from build123d import *

# Parameters (mm, degrees)
SKETCH1_W                = 60
SKETCH1_H                = 50
BOSS_EXTRUDE1_DEPTH      = 10
SKETCH3_W                = 50
SKETCH3_H                = 10
BOSS_EXTRUDE2_DEPTH      = 20
SKETCH2_W                = 20
SKETCH2_H                = 9
CUT_EXTRUDE2_DEPTH       = 2
SKETCH5_W                = 9
SKETCH5_H                = 20.5
CUT_EXTRUDE3_DEPTH       = 2
SKETCH6_R                = 0.75
CUT_EXTRUDE4_DEPTH       = 9
SKETCH9_W                = 10
SKETCH9_H                = 50
BOSS_EXTRUDE3_DEPTH      = 80
FILLET1_R                = 10
FILLET2_R                = 10
FILLET3_R                = 10
FILLET4_R                = 10
FILLET5_R                = 10
SKETCH11_W               = 10.5
SKETCH11_H               = 41
CUT_EXTRUDE5_DEPTH       = 40
SKETCH13_R               = 2
CUT_EXTRUDE6_DEPTH       = 40
MIRROR11_COPY_1_SKETCH_R = 2
MIRROR11_COPY_1_DEPTH    = 40


with BuildPart() as part:
    # Sketch1 → Boss-Extrude1 (new body)
    with BuildSketch(Plane(origin=(0, 0, 0), x_dir=(1, 0, 0), z_dir=(0, 1, 0))):
        with Locations((8.551590838, -18.42193)):
            Rectangle(SKETCH1_W, SKETCH1_H)
    extrude(amount=BOSS_EXTRUDE1_DEPTH)

    # Sketch3 → Boss-Extrude2 (add)
    with BuildSketch(Plane.ZY.offset(21.448409162)):
        with Locations((18.42193, 5)):
            Rectangle(SKETCH3_W, SKETCH3_H)
    extrude(amount=BOSS_EXTRUDE2_DEPTH)

    # Sketch2 → Cut-Extrude2 (cut)
    with BuildSketch(Plane(origin=(0, 10, 0), x_dir=(1, 0, 0), z_dir=(0, 1, 0))):
        with Locations((-18.948409162, -18.42193)):
            Rectangle(SKETCH2_W, SKETCH2_H)
    cut_extrude2 = extrude(amount=-CUT_EXTRUDE2_DEPTH, mode=Mode.SUBTRACT)

    # Mirror6: Cut-Extrude2 across plane
    add(cut_extrude2.mirror(Plane(origin=(-8.948409162, 8, 22.92193), x_dir=(0, 0, 1), z_dir=(1, 0, 0))), mode=Mode.SUBTRACT)

    # Sketch5 → Cut-Extrude3 (cut)
    with BuildSketch(Plane(origin=(0, 10, 0), x_dir=(1, 0, 0), z_dir=(0, 1, 0))):
        with Locations((-8.948409162, -3.67193)):
            Rectangle(SKETCH5_W, SKETCH5_H)
    cut_extrude3 = extrude(amount=-CUT_EXTRUDE3_DEPTH, mode=Mode.SUBTRACT)

    # Mirror7: Cut-Extrude3 across plane
    add(cut_extrude3.mirror(Plane.XY.offset(18.42193)), mode=Mode.SUBTRACT)

    # Sketch6 → Cut-Extrude4 (cut, through all)
    with BuildSketch(Plane(origin=(0, 8, 0), x_dir=(1, 0, 0), z_dir=(0, 1, 0))):
        with Locations((-25.448409162, -18.42193)):
            Circle(SKETCH6_R)
    cut_extrude4 = extrude(amount=-CUT_EXTRUDE4_DEPTH, mode=Mode.SUBTRACT)

    # Mirror8: Cut-Extrude4 across plane
    add(cut_extrude4.mirror(Plane(origin=(-8.948409162, 0, 0), x_dir=(0, 0, 1), z_dir=(1, 0, 0))), mode=Mode.SUBTRACT)

    # Sketch9 → Boss-Extrude3 (add)
    with BuildSketch(Plane(origin=(0, 10, 0), x_dir=(1, 0, 0), z_dir=(0, 1, 0))):
        with Locations((43.551590838, -18.42193)):
            Rectangle(SKETCH9_W, SKETCH9_H)
    extrude(amount=-BOSS_EXTRUDE3_DEPTH)

    # Fillet1
    fillet1_edges = [part.edges().sort_by_distance(p)[0] for p in [
        (48.551590838, 10, 18.42193),
    ]]
    fillet(fillet1_edges, radius=FILLET1_R)

    # Fillet2
    fillet2_edges = [part.edges().sort_by_distance(p)[0] for p in [
        (-41.448409162, 5, -6.57807),
    ]]
    fillet(fillet2_edges, radius=FILLET2_R)

    # Fillet3
    fillet3_edges = [part.edges().sort_by_distance(p)[0] for p in [
        (-41.448409162, 5, 43.42193),
    ]]
    fillet(fillet3_edges, radius=FILLET3_R)

    # Fillet4
    fillet4_edges = [part.edges().sort_by_distance(p)[0] for p in [
        (43.551590838, -70, 43.42193),
    ]]
    fillet(fillet4_edges, radius=FILLET4_R)

    # Fillet5
    fillet5_edges = [part.edges().sort_by_distance(p)[0] for p in [
        (43.551590838, -70, -6.57807),
    ]]
    fillet(fillet5_edges, radius=FILLET5_R)

    # Sketch11 → Cut-Extrude5 (cut)
    with BuildSketch(Plane.ZY.offset(-38.551590838)):
        with Locations((13.17193, -39.5)):
            Rectangle(SKETCH11_W, SKETCH11_H)
    cut_extrude5 = extrude(amount=-CUT_EXTRUDE5_DEPTH, mode=Mode.SUBTRACT)

    # Mirror9: Cut-Extrude5 across plane
    add(cut_extrude5.mirror(Plane(origin=(78.551590838, -60, 18.42193), x_dir=(1, 0, 0), z_dir=(0, 0, 1))), mode=Mode.SUBTRACT)

    # Sketch13 → Cut-Extrude6 (cut)
    with BuildSketch(Plane.ZY.offset(-38.551590838)):
        with Locations((12.52193, -63.56)):
            Circle(SKETCH13_R)
    cut_extrude6 = extrude(amount=-CUT_EXTRUDE6_DEPTH, mode=Mode.SUBTRACT)

    # Mirror10: Cut-Extrude6 across plane
    add(cut_extrude6.mirror(Plane.XY.offset(18.42193)), mode=Mode.SUBTRACT)

    # Mirror11: Cut-Extrude6 across plane
    add(cut_extrude6.mirror(Plane.ZX.offset(-39.5)), mode=Mode.SUBTRACT)

    # Mirror11 copy 1 sketch → Mirror11 copy 1 (cut)
    with BuildSketch(Plane(origin=(38.551590838, -79, 36.84386), x_dir=(0, 0, -1), z_dir=(-1, 0, 0))):
        with Locations((12.52193, -63.56)):
            Circle(MIRROR11_COPY_1_SKETCH_R)
    extrude(amount=-MIRROR11_COPY_1_DEPTH, mode=Mode.SUBTRACT)


solid = part.part
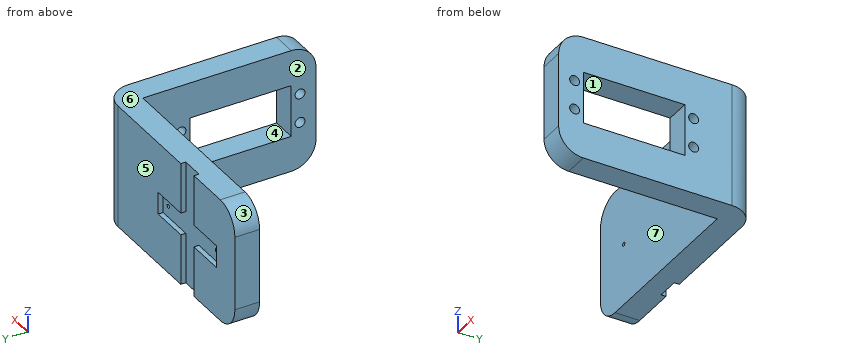
Work out the finished part from the listing and answer in its coordinate system (mm). Face numbers are marked on the shaded views. A direction names the side the tool comes from. Round coordinates to 2 decimals unless told otherwise and drop trailing zeros. Loops run counter-clockwise (first coordinate to the right, second up) from the corner with the lowest first, then second, coordinate; pieces in that order, holes last. Notation, with made-up numbers: (5.25, 37.5) -> (17.25, 37.5) arc R20 cw to (17.25, 55.5) -> close; hole circle Ø1 at (-15, 20.5). An arc over 180 degrees is marked (long way). Use one line per item in the form item = value.
(1) Flat-ended cylindrical pins translate along their axes: P1, Ø1, axis at y = 9.5, z = 35.5, coming from the +X side; P2, Ø0.9, axis at x = 7.55, z = 18.42, coming from the -Y side; P3, Ø2, axis at x = -32.5, z = -1, coming from the -Y side; P4, Ø6.5, axis at y = -15.44, z = 12.52, coming from the -X side. Find the tip coordinate at first contact, or state that the pin passes through.
Answer list:
P1 = 42.91
P2 = through
P3 = 0
P4 = 38.55
(2) Find section D-D on x = 28.5. Give the vertices of the cut face in (y, z), then the cut area to 3 significant figures.
Answer list:
outline = (0, -6.58) -> (10, -6.58) -> (10, 43.42) -> (0, 43.42) -> close
area = 500 mm2
(3) Straight lines are drawn through the part: line 1 (Y direction, x = 11, z = 23.5); line 2 (Z direction, x = 44, y = -15); line 3 (X direction, y = -38, z = 35). For each, find the intervals that lie inside material, in ascending order.
Answer list:
line_1 = 0 to 10
line_2 = -6.58 to 10.57, 14.47 to 22.37, 26.27 to 43.42
line_3 = 38.55 to 48.55
(4) Find section C-C on z = 5. Give the vertices of the cut face in (x, y).
Answer list:
outline = (-41.45, 0) -> (38.55, 0) -> (38.55, -70) -> (48.55, -70) -> (48.55, 0) arc R10 ccw to (38.55, 10) -> (-4.45, 10) -> (-4.45, 8) -> (-13.45, 8) -> (-13.45, 10) -> (-41.45, 10) -> close
(5) Find section A-A on y = -15.44. Give the vertices of the cut face in (x, z).
Answer list:
outline = (38.55, -6.58) -> (48.55, -6.58) -> (48.55, 10.52) -> (38.55, 10.52) -> close; (38.55, 14.52) -> (48.55, 14.52) -> (48.55, 22.32) -> (38.55, 22.32) -> close; (38.55, 26.32) -> (48.55, 26.32) -> (48.55, 43.42) -> (38.55, 43.42) -> close
(6) For a pull along Y with two mould halves and no side action, classify the marked faces 4, 5, 6 and 7 as released by +Y, released by -Y, zero draft, split by the parting line, or undercut.
Answer list:
face_4 = undercut
face_5 = released by +Y
face_6 = zero draft
face_7 = released by -Y
(7) Find section B-B on y = -41. Give the vertices of the cut face in (x, z), then the cut area to 3 significant figures.
Answer list:
outline = (38.55, -6.58) -> (48.55, -6.58) -> (48.55, 7.92) -> (38.55, 7.92) -> close; (38.55, 28.92) -> (48.55, 28.92) -> (48.55, 43.42) -> (38.55, 43.42) -> close
area = 290 mm2
(8) A tool of negligible diameter and unlimited length cuts with its end or side. For the marked faces 1, 2 and 3, from which of +Z, -Z, +X, -X, +Y, -Y can it reach the whole face along a straight path? Write none if from no direction.
Answer list:
face_1 = +X, -X
face_2 = +Z, -Z, -X, -Y
face_3 = +Z, -X, +Y, -Y
